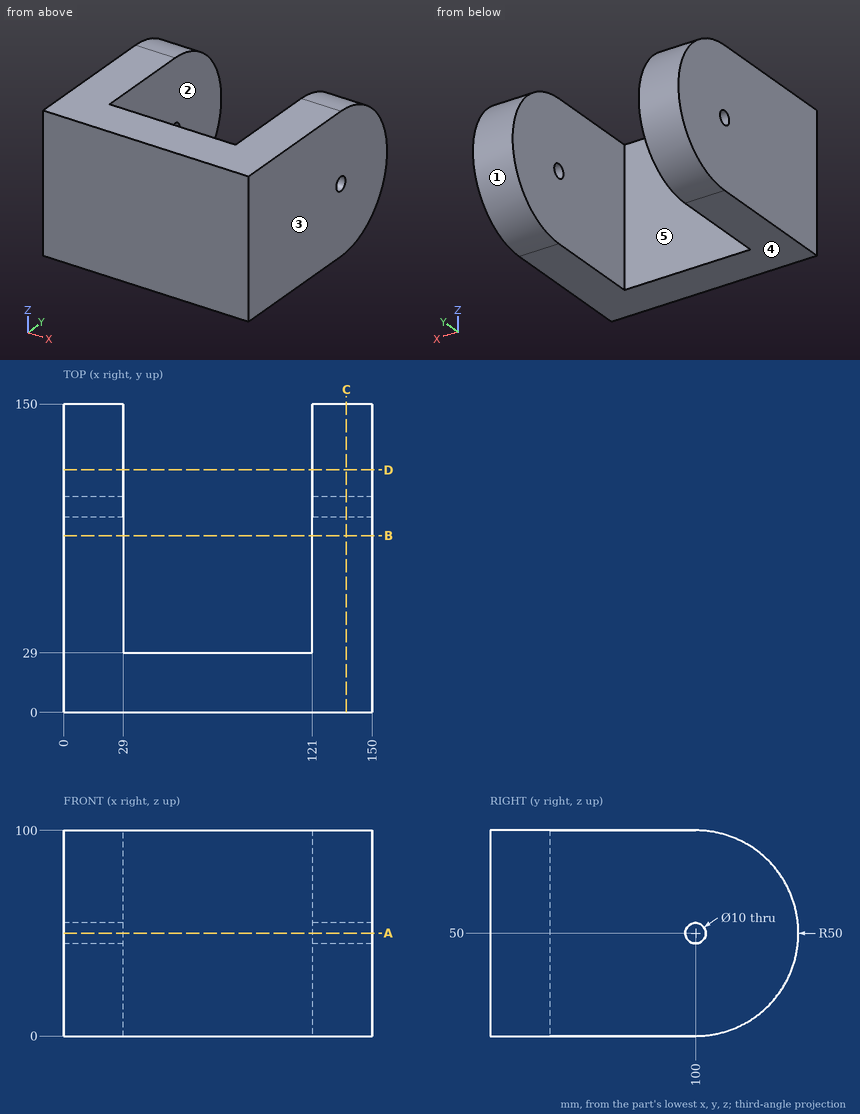
Check sheet for the drawn part. Datum: minimum x, y, z corner. Units: mm. A direction names the side the tool comes from. Coordinates: 2 decimals unless noted, no trailing zeros. Order: outer loops, then holes, each group sorted by start corner. A loop starts at its lowest first (then second) coordinate and runs counter-clockwise, first axis right, second up. Notation, with made-up numbers: (63.25, 73.25) - (110.25, 73.25) arc R17 cw to (110.25, 105.25) - close; hole circle Ø1 at (-34, 67). An arc over 180 degrees is marked (long way). Return JSON: item names as keys, results as strings.
(1) Section check B-B, the plane y = 86. Record the cut outline in (x, z), and give its area (3 significant figures).
Filled sheet:
{"outline": "(0, 0) - (29, 0) - (29, 100) - (0, 100) - close; (121, 0) - (150, 0) - (150, 100) - (121, 100) - close", "area": "5,800 mm^2"}
(2) Section check D-D, the plane y = 118. Record the cut outline in (x, z), and give its area (3 significant figures).
Filled sheet:
{"outline": "(0, 3.35) - (29, 3.35) - (29, 96.65) - (0, 96.65) - close; (121, 3.35) - (150, 3.35) - (150, 96.65) - (121, 96.65) - close", "area": "5,410 mm^2"}
(3) Section check C-C, the plane x = 137.5. Record the cut outline in (y, z).
Filled sheet:
{"outline": "(0, 0) - (100, 0) arc R50 ccw to (100, 100) - (0, 100) - close; hole circle Ø10 at (100, 50)"}
(4) Thickness scan on line 1 along X through (y, z) = (132, 82.5); line 2 along Z through (x, y) = (128, 100); line 3 along Y through (x, z) = (8.25, 50). Record the ranges inside material, lowest first.
Filled sheet:
{"line 1": "x = 0 to 29, 121 to 150", "line 2": "z = 0 to 45, 55 to 100", "line 3": "y = 0 to 95, 105 to 150"}
(5) Section check A-A, the plane z = 50. Record the cut outline in (x, y), and give its area (3 significant figures).
Filled sheet:
{"outline": "(0, 0) - (150, 0) - (150, 95) - (121, 95) - (121, 29) - (29, 29) - (29, 95) - (0, 95) - close; (0, 105) - (29, 105) - (29, 150) - (0, 150) - close; (121, 105) - (150, 105) - (150, 150) - (121, 150) - close", "area": "10,800 mm^2"}
(6) Go/stop test with flat-tipped pins: pin 1 (6 mm diameter, centred on x = 36.5, z = 89.5, fed in from -Y); pin 2 (12 mm diameter, centred on x = 88.5, z = 84.5, fed in from +Y). Record where each tip stops, or that it passes through.
Filled sheet:
{"pin 1": "stops at y = 0", "pin 2": "stops at y = 29"}
(7) Access from +Z, -Z, +X, -X, +Y, -Y to the whole of each face (thin tool, end or side, straight path). Record for the marked faces 1 and 2.
Filled sheet:
{"face 1": "+X, -X, +Y", "face 2": "+Z, -Z, +Y"}
(8) Mould release check, pull along X, two halves, no side actions. Record for the marked faces 3, 4 and 5: pulls with the +X half, pulls with the -X half, needs draft (parallel to the pull), parting line crosses it, or undercut.
Filled sheet:
{"face 3": "pulls with the +X half", "face 4": "needs draft", "face 5": "undercut"}
